from build123d import *

# Parameters (mm, degrees)
BOSS_EXTRU_1_DEPTH = 3


with BuildPart() as part:
    # Esquisse2 → Boss.-Extru.1 (new body)
    with BuildSketch(Plane(origin=(0, 0, -25.32076404), x_dir=(0, 0, -1), z_dir=(1, 0, 0))):
        with BuildLine():
            Line((-45.329923666, 87.110380525), (-45.329923666, 67.110380525))
            ThreePointArc((-45.329923666, 67.110380525), (-20.329923666, 55.930040637), (-45.329923666, 44.74970075))
            Line((-45.329923666, 44.74970075), (-45.329923666, -22.889619475))
            Line((-45.329923666, -22.889619475), (-35.329923666, -22.889619475))
            Line((-35.329923666, -22.889619475), (-35.329923666, 32.110380525))
            Line((-35.329923666, 32.110380525), (-30.329923666, 32.110380525))
            Line((-30.329923666, 32.110380525), (-30.329923666, -22.889619475))
            Line((-30.329923666, -22.889619475), (28.170076334, -22.889619475))
            Line((28.170076334, -22.889619475), (28.170076334, 32.110380525))
            Line((28.170076334, 32.110380525), (33.170076334, 32.110380525))
            Line((33.170076334, 32.110380525), (33.170076334, -22.889619475))
            Line((33.170076334, -22.889619475), (91.670076334, -22.889619475))
            Line((91.670076334, -22.889619475), (91.670076334, 32.110380525))
            Line((91.670076334, 32.110380525), (96.670076334, 32.110380525))
            Line((96.670076334, 32.110380525), (96.670076334, -22.889619475))
            Line((96.670076334, -22.889619475), (106.670076334, -22.889619475))
            Line((106.670076334, -22.889619475), (106.670076334, 44.74970075))
            ThreePointArc((106.670076334, 44.74970075), (131.670076334, 55.930040637), (106.670076334, 67.110380525))
            Line((106.670076334, 67.110380525), (106.670076334, 87.110380525))
            Line((106.670076334, 87.110380525), (-45.329923666, 87.110380525))
        make_face()
    extrude(amount=BOSS_EXTRU_1_DEPTH)


solid = part.part
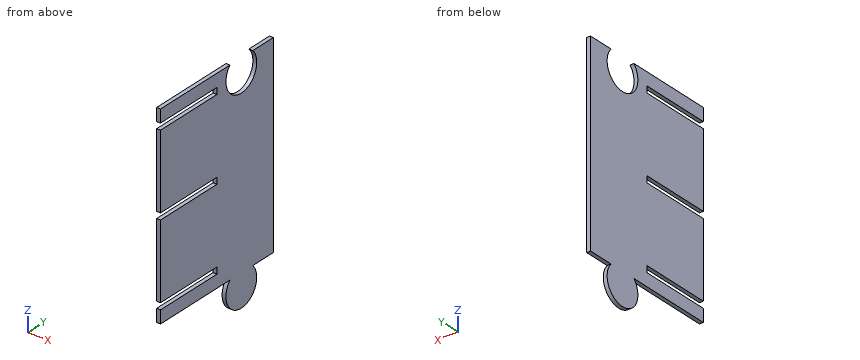
Verification items for the finished model (mm, model axes). Round coordinates to 2 decimals unless told otherwise and drop trailing zeros. Loops run counter-clockwise (first coordinate to the right, second up) from the corner with the lowest first, then second, coordinate; pieces in that order, holes last. Notation, with made-up numbers: (64, 28.5) - (96, 28.5) arc R13 ccw to (96, 40.5) - close; hole circle Ø1 at (27.25, 65.5). An arc over 180 degrees is marked (long way). Use a Markdown table: item, result. Add a question column.
1. Section check A-A, the plane y = 22.5. Record the boundary of the cut face in (x, z), plus the area to 3 significant figures.
2. Section check C-C, the plane y = 69. Record the boundary of the cut face in (x, z).
3. Section check B-B, the plane x = 0.5. Record the boundary of the cut face in (y, z).
4. Thickness scan on probe 1 along Z at (x, y) = (1.1, 9); probe 2 along Z at (x, y) = (2.85, 37); probe 3 along Y at (x, z) = (0.35, -142). Record the ranges inside material, lowest first. Write a range as [from, to].
5. Gauge pin test, flat ends, axial feed: pin 1 (1.5 mm diameter, centred on x = 1.5, z = -120, fed in from -Y); pin 2 (0.9 mm diameter, centred on x = 1, y = 3.5, fed in from -Z); pin 3 (24 mm diameter, centred on y = 55.93, z = 10.01, fed in from -X). Record the tip position at first contact, or that the pin passes through.
6. Section check D-D, the plane z = 1. Record the boundary of the cut face in (x, y), plus the area to 3 significant figures.
Checks:
| question | item | result |
|---|---|---|
| 1 | outline | (0, -131.99) - (3, -131.99) - (3, -121.99) - (0, -121.99) - close; (0, -116.99) - (3, -116.99) - (3, -58.49) - (0, -58.49) - close; (0, -53.49) - (3, -53.49) - (3, 5.01) - (0, 5.01) - close; (0, 10.01) - (3, 10.01) - (3, 20.01) - (0, 20.01) - close |
| 1 | area | 411 mm^2 |
| 2 | outline | (0, -149.35) - (3, -149.35) - (3, -134.63) - (0, -134.63) - close; (0, -131.99) - (3, -131.99) - (3, 2.65) - (0, 2.65) - close; (0, 17.37) - (3, 17.37) - (3, 20.01) - (0, 20.01) - close |
| 3 | outline | (-22.89, -131.99) - (44.75, -131.99) arc R15 ccw (long way) to (67.11, -131.99) - (87.11, -131.99) - (87.11, 20.01) - (67.11, 20.01) arc R15 cw (long way) to (44.75, 20.01) - (-22.89, 20.01) - (-22.89, 10.01) - (32.11, 10.01) - (32.11, 5.01) - (-22.89, 5.01) - (-22.89, -53.49) - (32.11, -53.49) - (32.11, -58.49) - (-22.89, -58.49) - (-22.89, -116.99) - (32.11, -116.99) - (32.11, -121.99) - (-22.89, -121.99) - close |
| 4 | probe 1 | z = [-131.99, -121.99], [-116.99, -58.49], [-53.49, 5.01], [10.01, 20.01] |
| 4 | probe 2 | z = [-131.99, 20.01] |
| 4 | probe 3 | y = [40.93, 70.93] |
| 5 | pin 1 | stops at y = 32.11 |
| 5 | pin 2 | stops at z = -131.99 |
| 5 | pin 3 | passes through |
| 6 | outline | (0, -22.89) - (3, -22.89) - (3, 43.94) - (0, 43.94) - close; (0, 67.92) - (3, 67.92) - (3, 87.11) - (0, 87.11) - close |
| 6 | area | 258 mm^2 |
